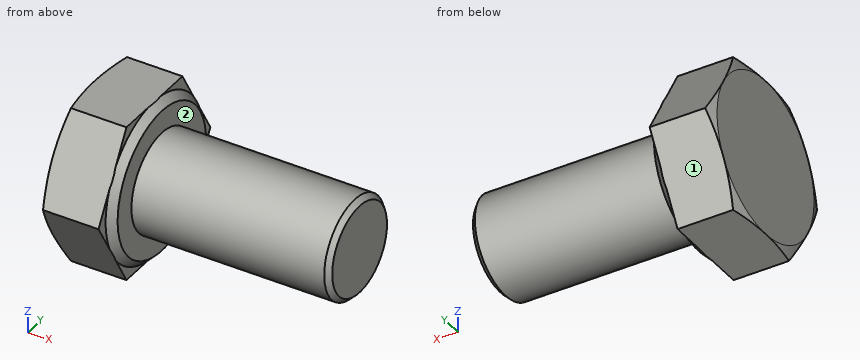
```python
from build123d import *

# Parameters (mm, degrees)
BASEHEAD_DEPTH = 5.45
SKETCH5_R      = 4
BASEBODY_DEPTH = 16


with BuildPart() as part:
    # Sketch2 → BaseHead (new body)
    with BuildSketch(Plane(origin=(0, 0, 0), x_dir=(0, 0, -1), z_dir=(1, 0, 0))):
        Polygon((6.365, -3.674834463), (6.365, 3.674834463), (0, 7.349668927), (-6.365, 3.674834463), (-6.365, -3.674834463), (0, -7.349668927), align=None)
    extrude(amount=BASEHEAD_DEPTH)

    # Sketch3 → BearingFace (revolve, cut)
    with BuildSketch(Plane.XY, mode=Mode.PRIVATE) as bearingface_sk:
        Polygon((5.45, 7.349668927), (5.45, 5.815), (4.85, 6.415), (4.85, 7.349668927), align=None)
    revolve(bearingface_sk.sketch.rotate(Axis((-0.957090588, 0, 0), (1, 0, 0)), 90), axis=Axis((-0.957090588, 0, 0), (1, 0, 0)), mode=Mode.SUBTRACT)

    # Sketch4 → HeadChamfer (revolve, cut)
    with BuildSketch(Plane.XY):
        Polygon((0, 7.349668927), (0.35839018, 7.349668927), (0, 6.365), align=None)
    revolve(axis=Axis((-0.493528746, 0, 0), (1, 0, 0)), mode=Mode.SUBTRACT)

    # Sketch5 → BaseBody (add)
    with BuildSketch(Plane(origin=(5.45, 0, 0), x_dir=(0, 0, -1), z_dir=(1, 0, 0))):
        Circle(SKETCH5_R)
    extrude(amount=BASEBODY_DEPTH)

    # Chamfer1: read off the stored shape, not the designer's step
    # Chamfer1 outline → Chamfer1 (revolve, cut)
    with BuildSketch(Plane.YX):
        Polygon((4, 21.45), (3.6, 21.45), (4, 21.05), align=None)
    revolve(axis=Axis((0, 0, 0), (1, 0, 0)), mode=Mode.SUBTRACT)


solid = part.part
```
Work out the finished part from the listing and answer in its coordinate system (mm). Face numbers are marked on the shaded views. A direction names the side the tool comes from. Coordinates: 2 decimals unless noted, no trailing zeros. Write each loop counter-clockwise with the first axis right and the second up, starting at its lowest first coordinate (ties: lowest second). Pieces come first, ordered by that corner, then holes.
Q1. Find the intervals of material crossed by line 1 (X direction, y = 5, z = -1.75); line 2 (Z direction, x = 17.75, y = 0); line 3 (Y direction, x = 20, z = -2.5), in increasing order.
Q2. A cutting plane is placed at A-A, the plane x = 5.75. Give the vertices of the cut face in (y, z).
Q3. Each of these flat-tipped pins is pushed along its axis until it touches: pin 1 Ø1 at (y, z) = (-5, -4) entering from +X; pin 2 Ø1.5 at (x, y) = (7, -2.5) entering from -Z; pin 3 Ø1.2 at (y, z) = (-4, 5.5) entering from +X. Where does it stop, or does it pass through?
Q4. Which of the six approach directions +Z, -Z, +X, -X, +Y, -Y give full straight-line access (tool end or side, diameter ignored) to the marked faces 1 and 2?
Findings below:
1. line 1: x = 0 to 5.45
1. line 2: z = -4 to 4
1. line 3: y = -3.12 to 3.12
2. outline: circle Ø8 at (0, 0)
3. pin 1: stops at x = 5.36
3. pin 2: stops at z = -3.6
3. pin 3: stops at x = 5.06
4. face 1: -Z, +X, -X, +Y
4. face 2: +X
